Design review of the part built by this model. Coordinates are the model's own, in mm. A direction names the side the tool comes from. Coordinates: 2 decimals unless noted, no trailing zeros. Loops run counter-clockwise (first coordinate to the right, second up) from the corner with the lowest first, then second, coordinate; pieces in that order, holes last. Notation, with made-up numbers: (12.25, 44) -> (20.25, 44) arc R15 ccw to (20.25, 54) -> close; hole circle Ø6 at (67.25, -0.75). An arc over 180 degrees is marked (long way). Use one line per item in the form item = value. Start each with the question number.
1. Consider section A-A (z = 0). State the section outline as (x, y) points, then the cut area to 4 significant figures.
2. Consider section C-C (y = 4.5). State the section outline as (x, z) points.
3. Machinability: for faces 4 (the face through (-12.6, 5.11, 16.14)), 5 (the face through (-9.517, 2.532, -20.647)), 6 (the face through (3.89, 1.82, 20.65)), 7 (the face through (-2.36, 5.87, -19.4)), 8 (the face through (8.539, 1.972, 6.786)), which of the approach directions +Z, -Z, +X, -X, +Y, -Y give a long, thin tool a straight path to every point of the face, cutting with its end or side? Answer none if there is none.
4. Consider section D-D (z = -11). State the section outline as (x, y) points.
5. Consider section B-B (x = 0). State the section outline as (y, z) points.
6. Wall thickness on line 1 (Z direction, x = -5.25, y = 4.5); line 2 (X direction, y = 1.65, z = -11); line 3 (X direction, y = 4.25, z = 5): over which ranges is each line inside the solid? List them lowest first. Write a range as from..to.
7. For pin 1 (3 mm diameter, centred on x = 0, z = -11, fed in from -Y); pin 2 (3 mm diameter, centred on x = 0, z = 11, fed in from +Y); pin 3 (1.6 mm diameter, centred on x = -3.5, y = 2.75, fed in from -Z), all flat-tipped, find the tip position at first contact; note any pin that passes through.
8. The part is to be moulded in two halves that separate along Y. For faces 1 (the face through (0, 0, 6)), 2 (the face through (-10.45, 2.92, -16.4)), 3 (the face through (2.36, 5.87, 19.4)), say which applies: released by +Y, released by -Y, zero draft, split by the parting line, or undercut.
Autodesk Inventor part; units mm, degrees
ref_plane "YZ Plane" through (0, 0, 0) normal (1, 0, 0) x (0, 1, 0)
ref_plane "XZ Plane" through (0, 0, 0) normal (0, 1, 0) x (-1, 0, 0)
ref_plane "XY Plane" through (0, 0, 0) normal (0, 0, 1) x (1, 0, 0)
sketch "Sketch1" plane through (0, 0, 0) normal (0, 1, 0) x (-1, 0, 0)
  line L0 (15, 24.5) -> (-15, 24.5)
  line L1 (-15, 24.5) -> (-15, -24.5)
  line L2 (-15, -24.5) -> (15, -24.5)
  line L3 (15, -24.5) -> (15, 24.5)
  line L4 (0, 24.5) -> (0, -24.5) construction
  line L5 (15, 0) -> (-15, 0) construction
  line L6 (15, 0) -> (-15, 0) construction
  point P0 (0, 0)
  point P1 (0, 0)
  dimension "d0" = 49
  dimension "d1" = 30
  dimension "d64" = 0
extrude "Extrusion1" add sketch "Sketch1" along normal blind 6.25
sketch "Sketch2" plane through (0, 6.25, 0) normal (0, 1, 0) x (1, 0, 0)
  circle A0 centre (0, 0) radius 11 construction
  line L0 (0, 0) -> (-26.8985, 0) construction
  line L1 (-35.2782, 0) -> (23.3797, 0) construction
  point P0 (-14.9902, 25)
  point P1 (-11, 0)
  point P2 (-7.7782, -7.7782)
  point P3 (0, -11)
  point P4 (7.7782, -7.7782)
  point P5 (11, 0)
  point P6 (7.7782, 7.7782)
  point P7 (0, 11)
  point P8 (-7.7782, 7.7782)
  dimension "d7" = 22
  dimension "d8" = 360
hole "Hole1" at (-11, 6.25, 0) at (-7.7782, 6.25, -7.7782) at (0, 6.25, -11) at (7.7782, 6.25, -7.7782) at (11, 6.25, 0) at (7.7782, 6.25, 7.7782) at (0, 6.25, 11) at (-7.7782, 6.25, 7.7782) direction (0, -1, 0) diameter 2.5 end through all
sketch "Sketch3" plane through (0, 6.25, 0) normal (0, 1, 0) x (1, 0, 0)
  circle A0 centre (0, 0) radius 5.05
  dimension "d17" = 10.1
extrude "Extrusion2" cut sketch "Sketch3" against normal through all
sketch "Sketch6" plane through (-15, 0, 24.5) normal (0, 0, 1) x (1, 0, 0)
  line L0 (-10.3797, 2.75) -> (37.9037, 2.75) construction
  line L1 (0, 0) -> (30, 0) construction
  line L2 (0, 0) -> (0, 6.25)
  point P0 (15, 0)
  point P1 (4.5, 2.75)
  point P2 (11.5, 2.75)
  point P3 (18.5, 2.75)
  point P4 (25.5, 2.75)
  dimension "d33" = 2.75
  dimension "d34" = 4.5
  dimension "d37" = 7
hole "Hole3" at (-10.5, 2.75, 24.5) at (-3.5, 2.75, 24.5) at (3.5, 2.75, 24.5) at (10.5, 2.75, 24.5) direction (0, 0, -1) diameter 2.013 depth 7.6 tip angle 118
sketch "Sketch7" plane through (15, 0, -24.5) normal (0, 0, -1) x (-1, 0, 0)
  line L0 (-10.51, 2.75) -> (37.7733, 2.75) construction
  line L1 (0, 0) -> (29.8697, 0) construction
  line L2 (0, 0) -> (0, 3.7534)
  line L3 (0, 0) -> (30, 0)
  line L4 (0, 0) -> (0, 6.25)
  point P0 (15, 0)
  point P1 (15, 0)
  point P2 (4.5, 2.75)
  point P3 (11.5, 2.75)
  point P4 (18.5, 2.75)
  point P5 (25.5, 2.75)
  dimension "d53" = 2.75
  dimension "d54" = 4.5
  dimension "d55" = 7
hole "Hole4" at (10.5, 2.75, -24.5) at (-10.5, 2.75, -24.5) at (-3.5, 2.75, -24.5) at (3.5, 2.75, -24.5) direction (0, 0, 1) diameter 2.013 depth 7.6 tip angle 118
sketch "Sketch8" plane through (0, 6.25, 0) normal (0, 1, 0) x (1, 0, 0)
  line L0 (0, 35.3) -> (0, -40.3) construction
  line L1 (-15, -24.5) -> (15, -24.5)
  line L2 (15, 24.5) -> (-15, 24.5)
  line L3 (-1.5, -24.5) -> (-15, -24.5)
  line L4 (-15, -24.5) -> (-15, -18.5)
  line L5 (-15, -18.5) -> (-1.5, -18.5)
  line L6 (1.5, -24.5) -> (15, -24.5)
  line L7 (15, -24.5) -> (15, -18.5)
  line L8 (15, -18.5) -> (1.5, -18.5)
  line L9 (15, -24.5) -> (15, 24.5)
  line L10 (-15, 24.5) -> (-15, -24.5)
  line L11 (-1.5, -18.5) -> (-1.5, -24.5)
  line L12 (-15, -24.5) -> (15, -24.5)
  line L13 (1.5, -18.5) -> (1.5, -24.5)
  line L14 (-15, 0) -> (15, 0) construction
  line L15 (-1.5, 24.5) -> (-15, 24.5)
  line L16 (-15, 24.5) -> (-15, 18.5)
  line L17 (-15, 18.5) -> (-1.5, 18.5)
  line L18 (1.5, 24.5) -> (15, 24.5)
  line L19 (15, 24.5) -> (15, 18.5)
  line L20 (15, 18.5) -> (1.5, 18.5)
  line L21 (-1.5, 18.5) -> (-1.5, 24.5)
  line L22 (1.5, 18.5) -> (1.5, 24.5)
  line L23 (-15, -22.5) -> (15, -22.5) construction
  point P0 (0, 0)
  dimension "d80" = 6
  dimension "d81" = 3
  dimension "d82" = 13.5
  dimension "d86" = 2
extrude "Extrusion6" cut sketch "Sketch8" against normal blind 0.75 contours L4 L5 L11 L1 | L13 L8 L7 L1 | L10 L2 L21 L17 | L20 L22 L2 L9
fillet "Fillet1" radius 3 4 edges at (1.5, 5.875, 18.5) (-1.5, 5.875, 18.5) (1.5, 5.875, -18.5) (-1.5, 5.875, -18.5)
sketch "Sketch11" plane through (0, 6.25, 0) normal (0, 1, 0) x (1, 0, 0)
  line L0 (-13.5, -17) -> (13.5, -17)
  line L1 (13.5, -17) -> (13.5, 17)
  line L2 (13.5, 17) -> (-13.5, 17)
  line L3 (-13.5, 17) -> (-13.5, -17)
  line L4 (-15, 18.5) -> (-15, -18.5)
  line L5 (15, -18.5) -> (15, 18.5)
  line L6 (-1.5, -24.5) -> (-15, -24.5)
  line L7 (-15, 24.5) -> (-1.5, 24.5)
  point P0 (0, 0)
  dimension "d87" = 7.5
  dimension "d88" = 7.5
  dimension "d91" = 1.5
  dimension "d92" = 1.5
extrude "Extrusion7" cut sketch "Sketch11" against normal blind 2.25
fillet "Fillet2" radius 3 4 edges at (-13.5, 5.125, 17) (13.5, 5.125, 17) (13.5, 5.125, -17) (-13.5, 5.125, -17)
equation "\"d3\" = thickness"
equation "\"d7\" = d9"
equation "\"d18\" = thickness"
equation "\"d33\" = hole_2_bottom"
equation "\"d53\" = hole_2_bottom"
equation "\"d83\" = thickness - border_thickness"
equation "\"d89\" = thickness - central_thickness"
equation "\"thickness\" = 6.25"
equation "\"d9\" = 22"
equation "\"tol\" = 0.1"
equation "\"border_thickness\" = 5.5"
equation "\"central_thickness\" = 4"
equation "\"hole_2_bottom\" = 0.5 * border_thickness"
properties part number "new_base_u64_long" material "Aluminum 2014-T4"
Geometry check:
q1.outline = (-15, 0) -> (-12.25, 0) -> (-12.25, 4) -> (-13.5, 4) -> (-13.5, 6.25) -> (-15, 6.25) -> close; (-9.75, 0) -> (-5.05, 0) -> (-5.05, 4) -> (-9.75, 4) -> close; (5.05, 0) -> (9.75, 0) -> (9.75, 4) -> (5.05, 4) -> close; (12.25, 0) -> (15, 0) -> (15, 6.25) -> (13.5, 6.25) -> (13.5, 4) -> (12.25, 4) -> close
q1.area = 66.35 mm²
q2.outline = (-15, -24.5) -> (15, -24.5) -> (15, 24.5) -> (-15, 24.5) -> close; hole (-13.5, -14) arc R3 ccw to (-10.5, -17) -> (10.5, -17) arc R3 ccw to (13.5, -14) -> (13.5, 14) arc R3 ccw to (10.5, 17) -> (-10.5, 17) arc R3 ccw to (-13.5, 14) -> close
q3.face_4 = +Y
q3.face_5 = -Z
q3.face_6 = +Z
q3.face_7 = -Z, -X, +Y
q3.face_8 = +Y, -Y
q4.outline = (-15, 0) -> (-1.25, 0) -> (-1.25, 4) -> (-13.5, 4) -> (-13.5, 6.25) -> (-15, 6.25) -> close; (1.25, 0) -> (15, 0) -> (15, 6.25) -> (13.5, 6.25) -> (13.5, 4) -> (1.25, 4) -> close
q5.outline = (0, -24.5) -> (6.25, -24.5) -> (6.25, -17) -> (4, -17) -> (4, -12.25) -> (0, -12.25) -> close; (0, -9.75) -> (4, -9.75) -> (4, -5.05) -> (0, -5.05) -> close; (0, 5.05) -> (4, 5.05) -> (4, 9.75) -> (0, 9.75) -> close; (0, 12.25) -> (4, 12.25) -> (4, 17) -> (6.25, 17) -> (6.25, 24.5) -> (0, 24.5) -> close
q6.line_1 = -24.5..-17, 17..24.5
q6.line_2 = -15..-1.25, 1.25..15
q6.line_3 = -15..-13.5, 13.5..15
q7.pin_1 = 0
q7.pin_2 = 4
q7.pin_3 = -16.78
q8.face_1 = released by -Y
q8.face_2 = undercut
q8.face_3 = zero draft
